The model under review builds one solid part; all positions refer to its coordinate system, in mm. A direction names the side the tool comes from. Give positions to 0.01 mm unless a question says otherwise; leave off trailing zeros. Loops run counter-clockwise (first coordinate to the right, second up) from the corner with the lowest first, then second, coordinate; pieces in that order, holes last. Notation, with made-up numbers: (55.5, 31) - (59.5, 31) arc R32 cw to (59.5, 67) - close; hole circle Ø10 at (1.25, -16). An arc over 180 degrees is marked (long way). Return JSON: item names as keys, results as strings. Group by question number.
from build123d import *

# Parameters (mm, degrees)
SKETCH_W        = 24
SKETCH_H        = 24
SKETCH_R        = 2.5
SKETCH_R_2      = 1.1
PAD_DEPTH       = 8
SKETCH001_R     = 3
POCKET_DEPTH    = 1
SKETCH002_R     = 3
POCKET001_DEPTH = 10
SKETCH003_R     = 3
POCKET002_DEPTH = 8
FILLET_R        = 4
SKETCH004_R     = 2.25
POCKET003_DEPTH = 2
SKETCH005_R     = 3
POCKET004_DEPTH = 1


with BuildPart() as part:
    # Sketch → Pad (new body)
    with BuildSketch(Plane.XY):
        Rectangle(SKETCH_W, SKETCH_H)
        with Locations((-8, 8)):
            Circle(SKETCH_R, mode=Mode.SUBTRACT)
        with Locations((8, 8)):
            Circle(SKETCH_R, mode=Mode.SUBTRACT)
        with Locations((-8, -8)):
            Circle(SKETCH_R, mode=Mode.SUBTRACT)
        with Locations((8, -8)):
            Circle(SKETCH_R, mode=Mode.SUBTRACT)
        with Locations((1, -6)):
            Circle(SKETCH_R_2, mode=Mode.SUBTRACT)
    extrude(amount=PAD_DEPTH)

    # Sketch001 (on Face10 of Pad) → Pocket (cut)
    with BuildSketch(Plane(origin=(0, 0, 0), x_dir=(1, 0, 0), z_dir=(0, 0, -1))):
        with Locations((-8, 8)):
            Circle(SKETCH001_R)
        with Locations((8, 8)):
            Circle(SKETCH001_R)
        with Locations((8, -8)):
            Circle(SKETCH001_R)
        with Locations((-8, -8)):
            Circle(SKETCH001_R)
    extrude(amount=-POCKET_DEPTH, mode=Mode.SUBTRACT)

    # Sketch002 (on Face6 of Pocket) → Pocket001 (cut)
    with BuildSketch(Plane.YZ.offset(12)):
        Circle(SKETCH002_R)
    extrude(amount=-POCKET001_DEPTH, mode=Mode.SUBTRACT)

    # Sketch003 (on Face4 of Pocket001) → Pocket002 (cut)
    with BuildSketch(Plane(origin=(0, 0, 0), x_dir=(1, 0, 0), z_dir=(0, 0, -1))):
        with Locations((2, 0)):
            Circle(SKETCH003_R)
    extrude(amount=-POCKET002_DEPTH, mode=Mode.SUBTRACT)

    # Fillet
    fillet_edges = [part.edges().sort_by_distance(p)[0] for p in [
        (12, 12, 4),
        (12, -12, 4),
        (-12, -12, 4),
        (-12, 12, 4),
    ]]
    fillet(fillet_edges, radius=FILLET_R)

    # Sketch004 (on Face5 of Fillet) → Pocket003 (cut)
    with BuildSketch(Plane.XY.offset(8)):
        with Locations((1, -6)):
            Circle(SKETCH004_R)
    extrude(amount=-POCKET003_DEPTH, mode=Mode.SUBTRACT)

    # Sketch005 (on Face5 of Pocket003) → Pocket004 (cut)
    with BuildSketch(Plane.XY.offset(8)):
        with Locations((8, 8)):
            Circle(SKETCH005_R)
        with Locations((-8, -8)):
            Circle(SKETCH005_R)
        with Locations((8, -8)):
            Circle(SKETCH005_R)
        with Locations((-8, 8)):
            Circle(SKETCH005_R)
    extrude(amount=-POCKET004_DEPTH, mode=Mode.SUBTRACT)


solid = part.part
Item 1: Tool access review of faces 1 (the face through (8, 0, 3)), 2 (the face through (6, 10, 7)), 3 (the face through (9.15, 5.78, 3.96)), 4 (the face through (-5.14, 7.1, 0.49)): name each direction out of +Z, -Z, +X, -X, +Y, -Y from which nothing blocks a thin tool from reaching the whole face with its end or side.
Item 2: For P1, Ø2.5, axis at x = 1, y = -6, coming from the +Z side, flat-tipped, find the tip position at first contact; note if it passes through.
Item 3: Take a section at A-A (x = -6.5). State the section outline as (y, z) points.
Item 4: For L1, parallel to Y at x = 8, z = 7.5; L2, parallel to Y at x = -8, z = 4.65; L3, parallel to X at y = -9, z = 5.75, list the stretches that pass through material, from the lowest coordinate up. Write a range as from..to.
Item 5: Take a section at B-B (y = 9.5). State the section outline as (x, z) points.
Item 6: Mouldability with a two-part tool opening along X and no side actions: class faces 5 (the face through (10.797, -10.859, 4.056)), 6 (the face through (0, 3, 8)), 7 (the face through (-5.14, -8.9, 0.49)) as +X half, -X half, draft (parallel to the pull), parting line (faces both ways), or undercut.
Item 7: Take a section at D-D (x = 1). State the section outline as (y, z) points, then the cut area to 3 significant figures.
Item 8: Take a section at C-C (z = 3.5). State the section outline as (x, y) points.
Check sheet entries:
{
 "1": {"face 1": "-Z, +X", "face 2": "+Z", "face 3": "+Z, -Z", "face 4": "-Z"},
 "2": {"P1": "stops at z = 6"},
 "3": {"outline": "(-12, 0) - (-10.6, 0) - (-10.6, 1) - (-10, 1) - (-10, 7) - (-10.6, 7) - (-10.6, 8) - (-12, 8) - close; (-6, 1) - (-5.4, 1) - (-5.4, 0) - (5.4, 0) - (5.4, 1) - (6, 1) - (6, 7) - (5.4, 7) - (5.4, 8) - (-5.4, 8) - (-5.4, 7) - (-6, 7) - close; (10, 1) - (10.6, 1) - (10.6, 0) - (12, 0) - (12, 8) - (10.6, 8) - (10.6, 7) - (10, 7) - close"},
 "4": {"L1": "y = -12..-11, -5..5, 11..12", "L2": "y = -12..-10.5, -5.5..5.5, 10.5..12", "L3": "x = -11.87..-10.29, -5.71..5.71, 10.29..11.87"},
 "5": {"outline": "(-11.71, 0) - (-10.6, 0) - (-10.6, 1) - (-10, 1) - (-10, 7) - (-10.6, 7) - (-10.6, 8) - (-11.71, 8) - close; (-6, 1) - (-5.4, 1) - (-5.4, 0) - (5.4, 0) - (5.4, 1) - (6, 1) - (6, 7) - (5.4, 7) - (5.4, 8) - (-5.4, 8) - (-5.4, 7) - (-6, 7) - close; (10, 1) - (10.6, 1) - (10.6, 0) - (11.71, 0) - (11.71, 8) - (10.6, 8) - (10.6, 7) - (10, 7) - close"},
 "6": {"face 5": "+X half", "face 6": "draft", "face 7": "undercut"},
 "7": {"outline": "(-12, 0) - (-7.1, 0) - (-7.1, 6) - (-8.25, 6) - (-8.25, 8) - (-12, 8) - close; (-4.9, 0) - (-2.83, 0) - (-2.83, 8) - (-3.75, 8) - (-3.75, 6) - (-4.9, 6) - close; (2.83, 0) - (12, 0) - (12, 8) - (2.83, 8) - close", "area": "125 mm^2"},
 "8": {"outline": "(-12, -8) arc R4 ccw to (-8, -12) - (8, -12) arc R4 ccw to (12, -8) - (12, 8) arc R4 ccw to (8, 12) - (-8, 12) arc R4 ccw to (-12, 8) - close; hole circle Ø5 at (-8, -8); hole circle Ø5 at (-8, 8); hole circle Ø6 at (2, 0); hole circle Ø2.2 at (1, -6); hole circle Ø5 at (8, -8); hole circle Ø5 at (8, 8)"}
}
